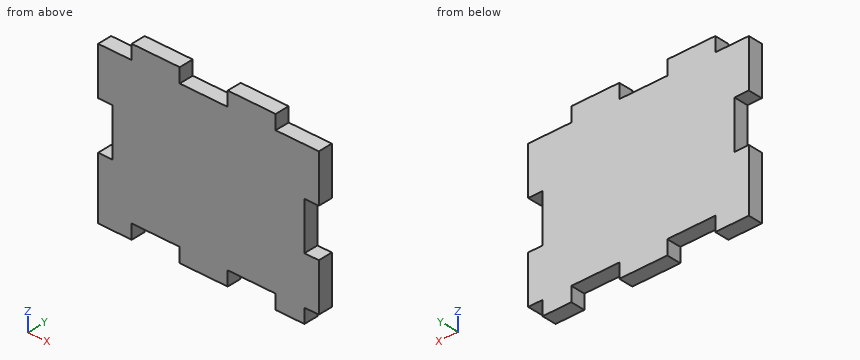
from build123d import *

# Parameters (mm, degrees)
RECTANGLE160_W                          = 3
RECTANGLE160_H                          = 10
EXTRUDE207_DEPTH                        = 3
EXTRUDE206_DEPTH                        = 3
RECTANGLE062_AS_DRAWN_W                 = 7
RECTANGLE062_AS_DRAWN_H                 = 3
EXTRUDE072_DEPTH                        = 3
EXTRUDE072_ONTO_RECTANGLE062_ROLL_ANGLE = 90
RECTANGLE060_AS_DRAWN_W                 = 10
RECTANGLE060_AS_DRAWN_H                 = 3
EXTRUDE070_DEPTH                        = 3
EXTRUDE070_ONTO_RECTANGLE060_ROLL_ANGLE = 90
RECTANGLE058_AS_DRAWN_W                 = 6
RECTANGLE058_AS_DRAWN_H                 = 3
EXTRUDE068_DEPTH                        = 3
EXTRUDE068_ONTO_RECTANGLE058_ROLL_ANGLE = 90
BOX006_W                                = 46
BOX006_H                                = 3
BOX006_DEPTH                            = 30
RECTANGLE067_AS_DRAWN_W                 = 10
RECTANGLE067_AS_DRAWN_H                 = 3
EXTRUDE077_DEPTH                        = 3
EXTRUDE077_ONTO_RECTANGLE067_ROLL_ANGLE = 90
RECTANGLE066_AS_DRAWN_W                 = 10
RECTANGLE066_AS_DRAWN_H                 = 3
EXTRUDE076_DEPTH                        = 3
EXTRUDE076_ONTO_RECTANGLE066_ROLL_ANGLE = 90


with BuildPart() as extrude207:
    # Rectangle160 → Extrude207 (new body)
    with BuildSketch(Plane(origin=(24, -68, 75), x_dir=(0, -1, 0), z_dir=(1, 0, 0))):
        with Locations((-1.5, 5)):
            Rectangle(RECTANGLE160_W, RECTANGLE160_H)
    extrude(amount=-EXTRUDE207_DEPTH)


with BuildPart() as extrude207_1:
    # Extrude207 placement: moved
    add(extrude207.part.moved(Location((-44, 0, 0))))


with BuildPart() as fusion064065:
    # Rectangle160 → Extrude206 (new body)
    with BuildSketch(Plane(origin=(24, -68, 75), x_dir=(0, -1, 0), z_dir=(1, 0, 0))):
        with Locations((-1.5, 5)):
            Rectangle(RECTANGLE160_W, RECTANGLE160_H)
    extrude(amount=-EXTRUDE206_DEPTH)


with BuildPart() as fusion064065_1:
    # Extrude206 placement: moved
    add(fusion064065.part.moved(Location((-1, 0, 0))))

    # Fusion064065: union Extrude207
    add(extrude207_1.part)


with BuildPart() as extrude072:
    # Rectangle062 as drawn → Extrude072 (new)
    with BuildSketch(Plane.XY):
        with Locations((-3.5, -1.5)):
            Rectangle(RECTANGLE062_AS_DRAWN_W, RECTANGLE062_AS_DRAWN_H)
    extrude(amount=-EXTRUDE072_DEPTH)


with BuildPart() as extrude072_1:
    # Extrude072 onto Rectangle062 roll: moved
    add(extrude072.part.rotate(Axis((0, 0, 0), (1, 0, 0)), EXTRUDE072_ONTO_RECTANGLE062_ROLL_ANGLE))


with BuildPart() as extrude072_2:
    # Extrude072 onto Rectangle062 placement: moved
    add(extrude072_1.part.moved(Location((-16, -68, 55))))


with BuildPart() as extrude070:
    # Rectangle060 as drawn → Extrude070 (new)
    with BuildSketch(Plane.XY):
        with Locations((-5, -1.5)):
            Rectangle(RECTANGLE060_AS_DRAWN_W, RECTANGLE060_AS_DRAWN_H)
    extrude(amount=-EXTRUDE070_DEPTH)


with BuildPart() as extrude070_1:
    # Extrude070 onto Rectangle060 roll: moved
    add(extrude070.part.rotate(Axis((0, 0, 0), (1, 0, 0)), EXTRUDE070_ONTO_RECTANGLE060_ROLL_ANGLE))


with BuildPart() as extrude070_2:
    # Extrude070 onto Rectangle060 placement: moved
    add(extrude070_1.part.moved(Location((4, -68, 55))))


with BuildPart() as finger_joints_aa:
    # Rectangle058 as drawn → Extrude068 (new)
    with BuildSketch(Plane.XY):
        with Locations((-3, -1.5)):
            Rectangle(RECTANGLE058_AS_DRAWN_W, RECTANGLE058_AS_DRAWN_H)
    extrude(amount=-EXTRUDE068_DEPTH)


with BuildPart() as finger_joints_aa_1:
    # Extrude068 onto Rectangle058 roll: moved
    add(finger_joints_aa.part.rotate(Axis((0, 0, 0), (1, 0, 0)), EXTRUDE068_ONTO_RECTANGLE058_ROLL_ANGLE))


with BuildPart() as finger_joints_aa_2:
    # Extrude068 onto Rectangle058 placement: moved
    add(finger_joints_aa_1.part.moved(Location((20, -68, 55))))

    # Fusion054: union Extrude072, Extrude070
    add(extrude072_2.part)
    add(extrude070_2.part)


with BuildPart() as obj1:
    # Box006 → Box006 (new body)
    with BuildSketch(Plane(origin=(-23, -68, 55), x_dir=(1, 0, 0), z_dir=(0, 0, 1))):
        with Locations((23, 1.5)):
            Rectangle(BOX006_W, BOX006_H)
    extrude(amount=BOX006_DEPTH)


with BuildPart() as obj2:
    # Rectangle067 as drawn → Extrude077 (new)
    with BuildSketch(Plane.XY):
        with Locations((-5, -1.5)):
            Rectangle(RECTANGLE067_AS_DRAWN_W, RECTANGLE067_AS_DRAWN_H)
    extrude(amount=-EXTRUDE077_DEPTH)


with BuildPart() as obj2_1:
    # Extrude077 onto Rectangle067 roll: moved
    add(obj2.part.rotate(Axis((0, 0, 0), (1, 0, 0)), EXTRUDE077_ONTO_RECTANGLE067_ROLL_ANGLE))


with BuildPart() as obj2_2:
    # Extrude077 onto Rectangle067 placement: moved
    add(obj2_1.part.moved(Location((-6, -68, 55))))


with BuildPart() as cut035055:
    # Rectangle066 as drawn → Extrude076 (new)
    with BuildSketch(Plane.XY):
        with Locations((-5, -1.5)):
            Rectangle(RECTANGLE066_AS_DRAWN_W, RECTANGLE066_AS_DRAWN_H)
    extrude(amount=-EXTRUDE076_DEPTH)


with BuildPart() as cut035055_1:
    # Extrude076 onto Rectangle066 roll: moved
    add(cut035055.part.rotate(Axis((0, 0, 0), (1, 0, 0)), EXTRUDE076_ONTO_RECTANGLE066_ROLL_ANGLE))


with BuildPart() as cut035055_2:
    # Extrude076 onto Rectangle066 placement: moved
    add(cut035055_1.part.moved(Location((14, -68, 55))))

    # Fusion057: union obj2
    add(obj2_2.part)


with BuildPart() as cut035055_3:
    # Fusion057 placement: moved
    add(cut035055_2.part.moved(Location((0, 0, 33))))

    # Fusion059: union Finger joints aa, obj1
    add(finger_joints_aa_2.part)
    add(obj1.part)

    # Cut035055: cut Fusion064065
    add(fusion064065_1.part, mode=Mode.SUBTRACT)


solid = cut035055_3.part
For this review, take the finished solid that the model builds, in its own axes (mm). Round coordinates to 2 decimals unless told otherwise and drop trailing zeros. Loops run counter-clockwise (first coordinate to the right, second up) from the corner with the lowest first, then second, coordinate; pieces in that order, holes last. Notation, with made-up numbers: (-32, 24) - (17, 24) arc R18 cw to (17, 49) - close; hole circle Ø11 at (44.5, -5). An arc over 180 degrees is marked (long way). Put each result on its own line as item: value. Start each with the question number.
1. For probe 1 along X at (y, z) = (-66.45, 85.5); probe 2 along X at (y, z) = (-67.65, 71); probe 3 along Z at (x, y) = (7.5, -65.8), list the stretches that pass through material, from the lowest coordinate up. Write a range as [from, to].
2. Insertion check: P1, Ø0.9, axis at x = 22, y = -66.5, coming from the -Z side; P2, Ø1.5, axis at x = -22, y = -67, coming from the +Z side; P3, Ø0.9, axis at y = -67, z = 54, coming from the +X side. Each pin has a flat end and moves straight along its axis. Give the tip position at first contact, or say it passes through.
3. Consider section D-D on z = 74. State the section outline as (x, y) points.
4. Consider section C-C on x = 4.5. State the section outline as (y, z) points, plus the area to 3 significant figures.
5. Consider section A-A on z = 85.5. State the section outline as (x, y) points, plus the area to 3 significant figures.
Result sheet:
1. probe 1: [-16, -6], [4, 14]
1. probe 2: [-20, 20]
1. probe 3: [55, 88]
2. P1: z = 55
2. P2: z = 85
2. P3: x = 20
3. outline: (-20, -68) - (20, -68) - (20, -65) - (-20, -65) - close
4. outline: (-68, 55) - (-65, 55) - (-65, 88) - (-68, 88) - close
4. area: 99.0 mm^2
5. outline: (-16, -68) - (-6, -68) - (-6, -65) - (-16, -65) - close; (4, -68) - (14, -68) - (14, -65) - (4, -65) - close
5. area: 60.0 mm^2
